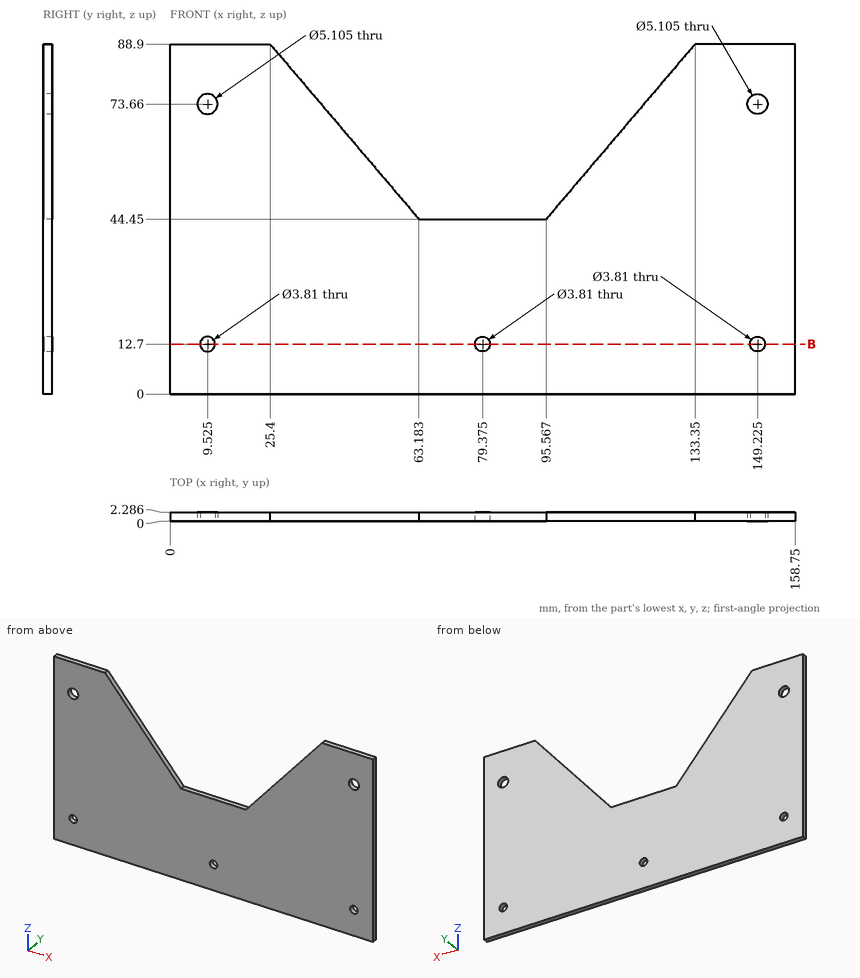
Input: dimensioned drawing with shaded views. Units: mm. Origin: part minimum x, y, z. Give positions to 0.01 mm unless a question says otherwise; leave off trailing zeros.
1. Section query B-B (z = 12.7). Count the separate pieces of the cut face and the enclosed holes in it.
2. First-contact query: pin 1 (0.7 mm diameter, centred on x = 83.5, y = 0.5, fed in from +Z). Flat tip, straight axial feed; report the tip coordinate or a pass-through.
3. Material intervals for line 1 along X through (y, z) = (0.6, 12.7); line 2 along Z through (x, y) = (86.5, 1.4); line 3 along Z through (x, y) = (40.5, 1.15) (1 decimal), sorted ascending.
Output values:
1. separate pieces: 4
1. enclosed holes: 0
2. pin 1: stops at z = 44.45
3. line 1: x = 0 to 7.62, 11.43 to 77.47, 81.28 to 147.32, 151.13 to 158.75
3. line 2: z = 0 to 44.45
3. line 3: z = 0 to 71.1
